from build123d import *

# Parameters (mm, degrees)
BOSS_EXTRUDE3_DEPTH           = 3.81
BOSS_EXTRUDE3_TAPER           = 9
BOSS_EXTRUDE3_OTHER_WAY_DEPTH = 3.81
BOSS_EXTRUDE3_OTHER_WAY_TAPER = 9
CUT_EXTRUDE1_DEPTH            = 1.778
CUT_EXTRUDE2_DEPTH            = 3.556
BOSS_EXTRUDE4_REACH           = 43.527
SKETCH6_R                     = 0.984091707
SKETCH7_W                     = 5.381079671
SKETCH7_H                     = 12.713539883
BOSS_EXTRUDE5_DEPTH           = 1.778


with BuildPart() as part:
    # Sketch1 → Boss-Extrude3 (new body)
    with BuildSketch(Plane.XY):
        with BuildLine():
            Line((-7.070417047, 6.599948555), (-4.176993685, -1.577117469))
            ThreePointArc((-4.176993685, -1.577117469), (0, -4.529882932), (4.176993685, -1.577117469))
            Line((4.176993685, -1.577117469), (7.070417047, 6.599948555))
            ThreePointArc((7.070417047, 6.599948555), (0, 16.601788433), (-7.070417047, 6.599948555))
        make_face()
    extrude(amount=BOSS_EXTRUDE3_DEPTH, taper=BOSS_EXTRUDE3_TAPER)

    # Sketch1 → Boss-Extrude3 other way (add)
    with BuildSketch(Plane.XY):
        with BuildLine():
            Line((-7.070417047, 6.599948555), (-4.176993685, -1.577117469))
            ThreePointArc((-4.176993685, -1.577117469), (0, -4.529882932), (4.176993685, -1.577117469))
            Line((4.176993685, -1.577117469), (7.070417047, 6.599948555))
            ThreePointArc((7.070417047, 6.599948555), (0, 16.601788433), (-7.070417047, 6.599948555))
        make_face()
    extrude(amount=-BOSS_EXTRUDE3_OTHER_WAY_DEPTH, taper=BOSS_EXTRUDE3_OTHER_WAY_TAPER)

    # Sketch3 → Cut-Extrude1 (cut)
    with BuildSketch(Plane.XY.offset(3.81)):
        with BuildLine():
            Line((-4.107021698, 7.648534601), (-1.213598336, -0.528531422))
            ThreePointArc((-1.213598336, -0.528531422), (0, -1.386438214), (1.213598336, -0.528531422))
            Line((1.213598336, -0.528531422), (4.107021698, 7.648534601))
            ThreePointArc((4.107021698, 7.648534601), (0, 13.458343715), (-4.107021698, 7.648534601))
        make_face()
    extrude(amount=-CUT_EXTRUDE1_DEPTH, mode=Mode.SUBTRACT)

    # Sketch4 → Cut-Extrude2 (cut)
    with BuildSketch(Plane.XY.offset(2.032)):
        with BuildLine():
            ThreePointArc((0.9304508, 6.328323332), (0, 12.801349411), (-0.9304508, 6.328323332))
            ThreePointArc((-0.9304508, 6.328323332), (0, 1.908170612), (0.9304508, 6.328323332))
        make_face()
    extrude(amount=-CUT_EXTRUDE2_DEPTH, mode=Mode.SUBTRACT)

    # Sketch6 → Boss-Extrude4 (add, up to next)
    with BuildSketch(Plane(origin=(0, -24.925590476, 0), x_dir=(1, 0, 0), z_dir=(0, 1, 0)), mode=Mode.PRIVATE) as boss_extrude4_sk1:
        Circle(SKETCH6_R)
    boss_extrude4_tool1 = extrude(boss_extrude4_sk1.sketch, amount=BOSS_EXTRUDE4_REACH, mode=Mode.PRIVATE) - part.part
    add(boss_extrude4_tool1.solids().sort_by_distance((0, -24.92559, 0))[0])

    # Sketch7 → Boss-Extrude5 (add, symmetric)
    with BuildSketch(Plane.XY):
        with Locations((0.003481044, -31.250797668)):
            Rectangle(SKETCH7_W, SKETCH7_H)
    extrude(amount=BOSS_EXTRUDE5_DEPTH, both=True)


solid = part.part
The listing builds one solid part. Answer for the finished solid, in the listing's coordinates (mm). A direction names the side the tool comes from. Give positions to 0.01 mm unless a question says otherwise; leave off trailing zeros. Write each loop counter-clockwise with the first axis right and the second up, starting at its lowest first coordinate (ties: lowest second). Pieces come first, ordered by that corner, then holes. Notation, with made-up numbers: (80.5, -39) -> (138.5, -39) arc R19 ccw to (138.5, -3) -> close; hole circle Ø10 at (-37, 67.5). An arc over 180 degrees is marked (long way). Use a Markdown table: item, result.
(1) Flat-ended cylindrical pins translate along their axes: P1, Ø1.1, axis at y = -29, z = 0, coming from the -X side; P2, Ø1.8, axis at x = 1, z = 0, coming from the +Y side; P3, Ø4, axis at y = -2.5, z = 0.5, coming from the +X side. Find the tip coordinate at first contact, or state that the pin passes through.
Return value:
| item | result |
|---|---|
| P1 | x = -2.69 |
| P2 | y = 16.6 |
| P3 | x = 4.54 |
(2) Section A-A, the plane z = 3 is taken. Determine the outline of the cut face in (x, y), then the cut area to 3 significant figures.
Return value:
| item | result |
|---|---|
| outline | (-6.62, 6.76) -> (-3.73, -1.42) arc R3.96 ccw to (3.73, -1.42) -> (6.62, 6.76) arc R7.02 ccw (long way) to start; hole (-4.11, 7.65) -> (-1.21, -0.53) arc R1.29 ccw to (1.21, -0.53) -> (4.11, 7.65) arc R4.36 ccw (long way) to start |
| area | 122 mm2 |
(3) Section D-D, the plane y = -14 is taken. Determine the outline of the cut face in (x, z), then the cut area to 3 significant figures.
Return value:
| item | result |
|---|---|
| outline | circle Ø1.97 at (0, 0) |
| area | 3.04 mm2 |
(4) Section C-C, the plane y = -28.5 is taken. Determine the outline of the cut face in (x, z), then the cut area to 3 significant figures.
Return value:
| item | result |
|---|---|
| outline | (-2.69, -1.78) -> (2.69, -1.78) -> (2.69, 1.78) -> (-2.69, 1.78) -> close |
| area | 19.1 mm2 |
(5) Determine the mould class of faces 1 (the flat face through (-2.68, 3.62, 2.93)), 2 (the flat face through (0, -31, -1.778)), 3 (the conical face through (0.191, 16.226, 2.355)) for opening direction X: released by +X, released by -X, zero draft, split by the parting line, or undercut.
Return value:
| item | result |
|---|---|
| face 1 | undercut |
| face 2 | zero draft |
| face 3 | split by the parting line |
(6) Section B-B, the plane x = 0 is taken. Determine the outline of the cut face in (y, z).
Return value:
| item | result |
|---|---|
| outline | (-37.61, -1.78) -> (-24.89, -1.78) -> (-24.89, -0.98) -> (-4.37, -0.98) -> (-3.93, -3.81) -> (16, -3.81) -> (16.6, 0) -> (16, 3.81) -> (13.46, 3.81) -> (13.46, 2.03) -> (12.8, 2.03) -> (12.8, -1.52) -> (1.91, -1.52) -> (1.91, 2.03) -> (-1.39, 2.03) -> (-1.39, 3.81) -> (-3.93, 3.81) -> (-4.37, 0.98) -> (-24.89, 0.98) -> (-24.89, 1.78) -> (-37.61, 1.78) -> close |
(7) For faces 4 (the cylindrical face through (-0.78, -14.77, 0.6)), 5 (the flat face through (2.694, -31, 0)), 6 (the flat face through (0, -31, 1.778)), 7 (the cylindrical face through (0.117, 13.457, 2.933)), determine the directions among +Z, -Z, +X, -X, +Y, -Y from which every point of the face is accessible in a straight line to the end or side of a thin tool.
Return value:
| item | result |
|---|---|
| face 4 | none |
| face 5 | +Z, -Z, +X, -Y |
| face 6 | +Z, +X, -X, -Y |
| face 7 | +Z |
(8) Find the intervals of material crossed by probe 1 along Y at (x, z) = (1.25, 1.25); probe 2 along Y at (x, z) = (-0.5, 0.5); probe 3 along Y at (x, z) = (1.5, 1.25), in increasing order. Write a range as from..to.
Return value:
| item | result |
|---|---|
| probe 1 | -37.61..-24.89, -4.14..2.28, 6.16..6.44, 12.56..16.3 |
| probe 2 | -37.61..1.96, 12.76..16.51 |
| probe 3 | -37.61..-24.89, -4.06..2.46, 5.97..6.55, 12.44..16.25 |
